from build123d import *

# Parameters (mm, degrees)
BASE_DEPTH        = 3.0988
SKETCH4_R         = 1.016
MOUNT_HOLES_DEPTH = 4.0988
EXTRUDE2_DEPTH    = 3.429
SKETCH3_W         = 8.382
SKETCH3_H         = 7.62
KEY_DEPTH         = 7.5278
KEYS_COUNT        = 4
KEYS_PITCH        = 14.14018
KEYS_COUNT_DIR2   = 4
KEYS_PITCH_DIR2   = 12.869418


with BuildPart() as part:
    # Sketch1 → base (new body)
    with BuildSketch(Plane.XY):
        with BuildLine():
            Line((-2.75, 38.75), (-33.5, 38.75))
            ThreePointArc((-33.5, 38.75), (-34.914213562, 38.164213562), (-35.5, 36.75))
            Line((-35.5, 36.75), (-35.5, -36.75))
            ThreePointArc((-35.5, -36.75), (-34.914213562, -38.164213562), (-33.5, -38.75))
            Line((-33.5, -38.75), (33.5, -38.75))
            ThreePointArc((33.5, -38.75), (34.914213562, -38.164213562), (35.5, -36.75))
            Line((35.5, -36.75), (35.5, 36.75))
            ThreePointArc((35.5, 36.75), (34.914213562, 38.164213562), (33.5, 38.75))
            Line((33.5, 38.75), (2.75, 38.75))
            Line((2.75, 38.75), (2.75, 35.75))
            Line((2.75, 35.75), (-2.75, 35.75))
            Line((-2.75, 35.75), (-2.75, 38.75))
        make_face()
    extrude(amount=BASE_DEPTH)

    # Sketch4 → mount holes (cut, through all)
    with BuildSketch(Plane.XY.offset(3.0988)):
        with Locations((-30, 29.5)):
            Circle(SKETCH4_R)
        with Locations((30, 29.5)):
            Circle(SKETCH4_R)
        with Locations((30, -29.5)):
            Circle(SKETCH4_R)
        with Locations((-30, -29.5)):
            Circle(SKETCH4_R)
    extrude(amount=-MOUNT_HOLES_DEPTH, mode=Mode.SUBTRACT)

    # Sketch2 → Extrude2 (add)
    with BuildSketch(Plane.XY.offset(3.0988)):
        with BuildLine():
            Line((-27.5, 34), (27.5, 34))
            ThreePointArc((27.5, 34), (30.328427125, 32.828427125), (31.5, 30))
            Line((31.5, 30), (31.5, -30))
            ThreePointArc((31.5, -30), (30.328427125, -32.828427125), (27.5, -34))
            Line((27.5, -34), (-27.5, -34))
            ThreePointArc((-27.5, -34), (-30.328427125, -32.828427125), (-31.5, -30))
            Line((-31.5, -30), (-31.5, 30))
            ThreePointArc((-31.5, 30), (-30.328427125, 32.828427125), (-27.5, 34))
        make_face()
    extrude(amount=EXTRUDE2_DEPTH)

    # Sketch3 → key (cut, through all)
    with BuildSketch(Plane.XY.offset(6.5278)):
        with Locations((-21.209, 19.304)):
            Rectangle(SKETCH3_W, SKETCH3_H)
    key = extrude(amount=-KEY_DEPTH, mode=Mode.SUBTRACT)

    # keys: key 4 × 4
    with Locations(*[(i * KEYS_PITCH, -j * KEYS_PITCH_DIR2, 0) for i in range(KEYS_COUNT) for j in range(KEYS_COUNT_DIR2) if (i, j) != (0, 0)]):
        add(key, mode=Mode.SUBTRACT)


solid = part.part
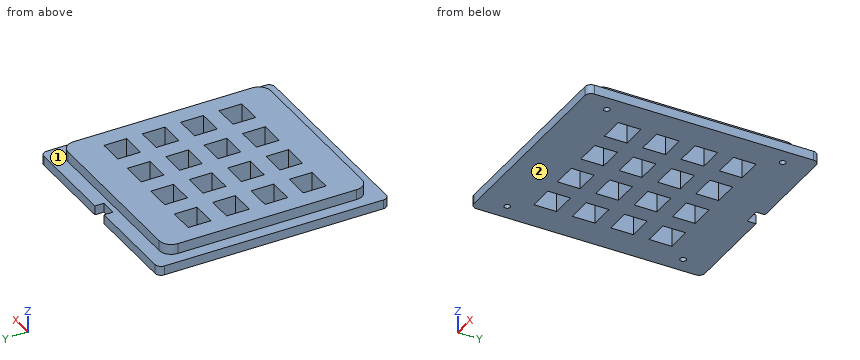
The listing builds one solid part. Answer for the finished solid, in the listing's coordinates (mm). Face numbers are marked on the shaded views. A direction names the side the tool comes from. Give positions to 0.01 mm unless a question says otherwise; leave off trailing zeros. Order: outer loops, then holes, each group sorted by start corner. A loop starts at its lowest first (then second) coordinate and runs counter-clockwise, first axis right, second up. Notation, with made-up numbers: (-13.75, -9.75) -> (15.25, -9.75) arc R24 ccw to (15.25, 14.25) -> close; hole circle Ø5 at (33.25, 63.5). An arc over 180 degrees is marked (long way). Put each result on its own line as item: value.
Item 1: A cutting plane is placed at A-A on y = 6. Give the vertices of the cut face in (x, z).
Established:
outline: (-35.5, 0) -> (-25.4, 0) -> (-25.4, 6.53) -> (-31.5, 6.53) -> (-31.5, 3.1) -> (-35.5, 3.1) -> close; (-17.02, 0) -> (-11.26, 0) -> (-11.26, 6.53) -> (-17.02, 6.53) -> close; (-2.88, 0) -> (2.88, 0) -> (2.88, 6.53) -> (-2.88, 6.53) -> close; (11.26, 0) -> (17.02, 0) -> (17.02, 6.53) -> (11.26, 6.53) -> close; (25.4, 0) -> (35.5, 0) -> (35.5, 3.1) -> (31.5, 3.1) -> (31.5, 6.53) -> (25.4, 6.53) -> close
Item 2: A cutting plane is placed at D-D on z = 1.5. Count the separate pieces of the cut face and the enclosed holes in it, plus the area to 3 significant figures.
Established:
separate pieces: 1
enclosed holes: 20
area: 4,450 mm^2
Item 3: Given P1, Ø2, axis at x = 6, z = 4.5, coming from the +Y side; P2, Ø3.5, axis at x = 23, z = 4, coming from the +Y side; P3, Ø1.5, axis at y = 20, z = 4, coming from the -X side; P4, Ø1, axis at x = 25, z = 5.5, coming from the -Y side, each flat-ended and moving along its own axis, determine where each tip first touches the part or whether it passes through.
Established:
P1: stops at y = 34
P2: stops at y = 38.75
P3: stops at x = -31.5
P4: stops at y = -34
Item 4: For the marked faces 1 and 2, determine the directions among +Z, -Z, +X, -X, +Y, -Y from which every point of the face is accessible in a straight line to the end or side of a thin tool.
Established:
face 1: +Z
face 2: -Z, +X, -X, +Y, -Y
Item 5: A cutting plane is placed at B-B on x = -23. Give the vertices of the cut face in (y, z).
Established:
outline: (-38.75, 0) -> (-23.11, 0) -> (-23.11, 6.53) -> (-34, 6.53) -> (-34, 3.1) -> (-38.75, 3.1) -> close; (-15.49, 0) -> (-10.24, 0) -> (-10.24, 6.53) -> (-15.49, 6.53) -> close; (-2.62, 0) -> (2.62, 0) -> (2.62, 6.53) -> (-2.62, 6.53) -> close; (10.24, 0) -> (15.49, 0) -> (15.49, 6.53) -> (10.24, 6.53) -> close; (23.11, 0) -> (38.75, 0) -> (38.75, 3.1) -> (34, 3.1) -> (34, 6.53) -> (23.11, 6.53) -> close
Item 6: A cutting plane is placed at C-C on x = -12.5. Give the vertices of the cut face in (y, z).
Established:
outline: (-38.75, 0) -> (38.75, 0) -> (38.75, 3.1) -> (34, 3.1) -> (34, 6.53) -> (-34, 6.53) -> (-34, 3.1) -> (-38.75, 3.1) -> close
Item 7: Straight lines are drawn through the part: line 1 (Y direction, x = 21, z = 3.75); line 2 (X direction, y = 3, z = 4.25); line 3 (Y direction, x = -18.5, z = 0.5). For each, find the intervals that lie inside material, in ascending order.
Established:
line 1: y = -34 to -23.11, -15.49 to -10.24, -2.62 to 2.62, 10.24 to 15.49, 23.11 to 34
line 2: x = -31.5 to -25.4, -17.02 to -11.26, -2.88 to 2.88, 11.26 to 17.02, 25.4 to 31.5
line 3: y = -38.75 to -23.11, -15.49 to -10.24, -2.62 to 2.62, 10.24 to 15.49, 23.11 to 38.75
